```python
from build123d import *

# Parameters (mm, degrees)
SKETCH_1_W          = 54
SKETCH_1_H          = 60
SKETCH_1_R          = 1.1
EXTRUDE_1_DEPTH     = 2.2
SKETCH_2_R          = 3
SKETCH_2_R_2        = 2.929560398
CUT_EXTRUDE_1_DEPTH = 0.8
SKETCH_3_R          = 1.1
SKETCH_3_R_2        = 1.55
CUT_EXTRUDE_2_DEPTH = 3.2
SKETCH_4_R          = 3.55
SKETCH_4_R_2        = 1.55
CUT_EXTRUDE_3_DEPTH = 0.8


with BuildPart() as part:
    # 草图1 → 凸台-拉伸1 (new body)
    with BuildSketch(Plane.XY):
        Rectangle(SKETCH_1_W, SKETCH_1_H)
        with Locations((-18, -25.8)):
            Circle(SKETCH_1_R, mode=Mode.SUBTRACT)
        with Locations((18, -25.8)):
            Circle(SKETCH_1_R, mode=Mode.SUBTRACT)
        with Locations((-18, 10.2)):
            Circle(SKETCH_1_R, mode=Mode.SUBTRACT)
        with Locations((18, 10.2)):
            Circle(SKETCH_1_R, mode=Mode.SUBTRACT)
    extrude(amount=EXTRUDE_1_DEPTH)

    # 草图2 → 切除-拉伸1 (cut)
    with BuildSketch(Plane(origin=(0, 0, 0), x_dir=(-1, 0, 0), z_dir=(0, 0, -1))):
        with Locations((-18, 10.2)):
            Circle(SKETCH_2_R)
        with Locations((18, 10.2)):
            Circle(SKETCH_2_R)
        with Locations((-18, -25.8)):
            Circle(SKETCH_2_R_2)
        with Locations((18, -25.8)):
            Circle(SKETCH_2_R)
    extrude(amount=-CUT_EXTRUDE_1_DEPTH, mode=Mode.SUBTRACT)

    # 草图3 → 切除-拉伸2 (cut, through all)
    with BuildSketch(Plane.XY.offset(2.2)):
        with Locations((-18, -25.8)):
            Circle(SKETCH_3_R)
        with Locations((-24, -26)):
            Circle(SKETCH_3_R_2)
        with Locations((-24, 26)):
            Circle(SKETCH_3_R_2)
        with Locations((24, -26)):
            Circle(SKETCH_3_R_2)
        with Locations((24, 26)):
            Circle(SKETCH_3_R_2)
    extrude(amount=-CUT_EXTRUDE_2_DEPTH, mode=Mode.SUBTRACT)

    # 草图4 → 切除-拉伸3 (cut)
    with BuildSketch(Plane(origin=(0, 0, 0), x_dir=(-1, 0, 0), z_dir=(0, 0, -1))):
        with Locations((-24, 26)):
            Circle(SKETCH_4_R)
        with Locations((-24, 26)):
            Circle(SKETCH_4_R_2, mode=Mode.SUBTRACT)
        with Locations((24, 26)):
            Circle(SKETCH_4_R)
        with Locations((24, 26)):
            Circle(SKETCH_4_R_2, mode=Mode.SUBTRACT)
        with Locations((24, -26)):
            Circle(SKETCH_4_R)
        with Locations((24, -26)):
            Circle(SKETCH_4_R_2, mode=Mode.SUBTRACT)
        with Locations((-24, -26)):
            Circle(SKETCH_4_R)
        with Locations((-24, -26)):
            Circle(SKETCH_4_R_2, mode=Mode.SUBTRACT)
    extrude(amount=-CUT_EXTRUDE_3_DEPTH, mode=Mode.SUBTRACT)


solid = part.part
```
Here's how the part is built. I have some questions about the finished solid (model axes, mm). A direction names the side the tool comes from. Coordinates: 2 decimals unless noted, no trailing zeros. Order: outer loops, then holes, each group sorted by start corner. A loop starts at its lowest first (then second) coordinate and runs counter-clockwise, first axis right, second up. Notation, with made-up numbers: (40, -36) - (63, -36) arc R16 ccw to (63, -8) - close; hole circle Ø9 at (86, -37.5). An arc over 180 degrees is marked (long way). One line per question, with ' | ' between items.
(1) Suppose I cut it at A-A on x = -18. List the corners of the cut face in (y, z) for me.
Report:
outline: (-30, 0) - (-28.8, 0) - (-28.8, 0.8) - (-26.9, 0.8) - (-26.9, 2.2) - (-30, 2.2) - close; (-24.7, 0.8) - (-22.8, 0.8) - (-22.8, 0) - (7.2, 0) - (7.2, 0.8) - (9.1, 0.8) - (9.1, 2.2) - (-24.7, 2.2) - close; (11.3, 0.8) - (13.2, 0.8) - (13.2, 0) - (30, 0) - (30, 2.2) - (11.3, 2.2) - close
(2) Will these pins go through, and if not, where does the flat tip stop? pin 1 (4 mm diameter, centred on x = 24, y = -26, fed in from -Z); pin 2 (1.3 mm diameter, centred on x = 18, y = 10.2, fed in from -Z).
Report:
pin 1: stops at z = 0.8 | pin 2: passes through
(3) Suppose I cut it at C-C on x = 24. List the corners of the cut face in (y, z) for me, and give its area (3 significant figures).
Report:
outline: (-30, 0) - (-29.55, 0) - (-29.55, 0.8) - (-27.55, 0.8) - (-27.55, 2.2) - (-30, 2.2) - close; (-24.45, 0.8) - (-22.45, 0.8) - (-22.45, 0) - (22.45, 0) - (22.45, 0.8) - (24.45, 0.8) - (24.45, 2.2) - (-24.45, 2.2) - close; (27.55, 0.8) - (29.55, 0.8) - (29.55, 0) - (30, 0) - (30, 2.2) - (27.55, 2.2) - close | area: 112 mm2
(4) If I drill on L1, parallel to Y at x = -18, z = 1.55; L2, parallel to Y at x = 24, z = 0.45; L3, parallel to X at y = 10.2, z = 1.45, over which ranges is the centre line in solid material (lowest first)?
Report:
L1: y = -30 to -26.9, -24.7 to 9.1, 11.3 to 30 | L2: y = -30 to -29.55, -22.45 to 22.45, 29.55 to 30 | L3: x = -27 to -19.1, -16.9 to 16.9, 19.1 to 27
(5) If we mould it in two halves opening along Y, with no side actions, what happens to faces 3 (the cylindrical face through (17.189, -25.057, 1.49)), 4 (the flat face through (22, 26, 0.8)), 5 (the flat face through (27, 0, 1))? For each: pulls with the +Y half, pulls with the -Y half, needs draft (parallel to the pull), parting line crosses it, or undercut.
Report:
face 3: undercut | face 4: undercut | face 5: needs draft
(6) For faces 1 (the cylindrical face through (-24.202, -24.463, 1.51)), 2 (the flat face through (-24, 28, 0.8)), which set-ups out of +Z, -Z, +X, -X, +Y, -Y let a thin tool reach every point of the face, with its end or its side?
Report:
face 1: +Z, -Z | face 2: -Z
(7) Suppose I cut it at B-B on y = 26. List the corners of the cut face in (x, z) for me.
Report:
outline: (-27, 0.8) - (-25.55, 0.8) - (-25.55, 2.2) - (-27, 2.2) - close; (-22.45, 0.8) - (-20.45, 0.8) - (-20.45, 0) - (20.45, 0) - (20.45, 0.8) - (22.45, 0.8) - (22.45, 2.2) - (-22.45, 2.2) - close; (25.55, 0.8) - (27, 0.8) - (27, 2.2) - (25.55, 2.2) - close
